Verification items for the finished model (mm, model axes). Face numbers are marked on the shaded views. A direction names the side the tool comes from. Coordinates: 2 decimals unless noted, no trailing zeros. Order: outer loops, then holes, each group sorted by start corner. A loop starts at its lowest first (then second) coordinate and runs counter-clockwise, first axis right, second up. Notation, with made-up numbers: (27, 25.5) -> (78, 25.5) arc R12 cw to (78, 32.5) -> close; hole circle Ø4 at (33, 19). An arc over 180 degrees is marked (long way). Write each question's results on one line, items separated by ' | '. Start each with the question number.
(1) Thickness scan on probe 1 along Z at (x, y) = (-0.5, -7); probe 2 along Y at (x, z) = (12.75, -7); probe 3 along Y at (x, z) = (1.25, -2). Record the ranges inside material, lowest first. Write a range as [from, to].
(2) Go/stop test with flat-tipped pins: pin 1 (1 mm diameter, centred on x = 9.5, y = -64, fed in from +Z); pin 2 (6 mm diameter, centred on x = 8.5, z = -6, fed in from +Y); pin 3 (3 mm diameter, centred on y = -14, z = 4, fed in from +X). Record where each tip stops, or that it passes through.
(3) Draft check along X on the marked faces 3, 4, 5 and 6. Enter one of: +X half, -X half, draft (parallel to the pull), parting line (faces both ways), or undercut.
(4) Set-up check for the marked faces 1 and 2: record each of +Z, -Z, +X, -X, +Y, -Y from which the full face is reachable in a straight line by a thin tool's end or side.
(5) Cross-section at A-A on y = 5.5. Enter the section's corners in (x, z), and give its area (3 significant figures).
(6) Cross-section at B-B on y = -47. Enter the section's corners in (x, z), and give its area (3 significant figures).
```python
from build123d import *

# Parameters (mm, degrees)
BOSS_EXTRUDE1_DEPTH = 12
SKETCH3_R           = 10
BOSS_EXTRUDE2_DEPTH = 75
CHAMFER1_SIZE       = 1


with BuildPart() as part:
    # Sketch1 → Boss-Extrude1 (new body)
    with BuildSketch(Plane(origin=(0, 0, 0), x_dir=(1, 0, 0), z_dir=(0, 1, 0))):
        Polygon((14, 8.082903769), (0, 16.165807537), (-14, 8.082903769), (-14, -8.082903769), (0, -16.165807537), (14, -8.082903769), align=None)
    extrude(amount=BOSS_EXTRUDE1_DEPTH)

    # Cut-Extrude1 cone 1 section (through the dimple's axis) → Cut-Extrude1 (revolve, cut)
    with BuildSketch(Plane(origin=(0, 12, 0), x_dir=(0, 0, 1), z_dir=(1, 0, 0))):
        Polygon((0, 0), (14, 0), (0, 8.082903769), align=None)
    revolve(axis=Axis((0, 12, 0), (0, -1, 0)), mode=Mode.SUBTRACT)

    # Sketch3 → Boss-Extrude2 (add)
    with BuildSketch(Plane.XZ):
        with Locations(Location((0, 0, 0), (0, 0, 270))):
            Circle(SKETCH3_R)
    extrude(amount=BOSS_EXTRUDE2_DEPTH)

    # Chamfer1
    chamfer1_edges = [part.edges().sort_by_distance(p)[0] for p in [
        (0, -75, 10),
    ]]
    chamfer(chamfer1_edges, length=CHAMFER1_SIZE)


solid = part.part
```
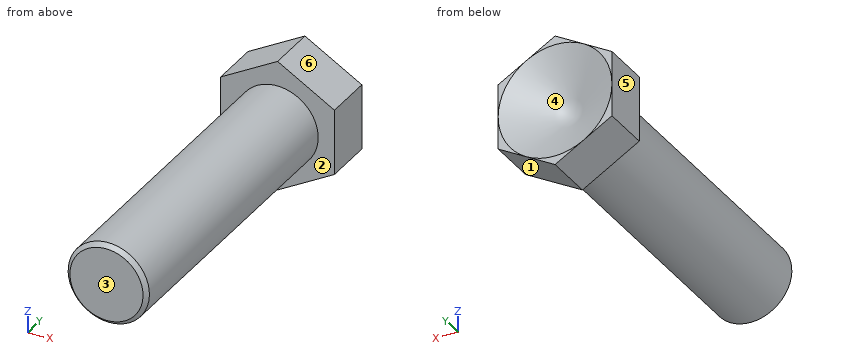
Results are:
1) probe 1: z = [-9.99, 9.99] | probe 2: y = [0, 12] | probe 3: y = [-75, 5.28]
2) pin 1: stops at z = 4.36 | pin 2: stops at y = 11.66 | pin 3: stops at x = 9.68
3) face 3: draft | face 4: undercut | face 5: -X half | face 6: +X half
4) face 1: -Z, +X, +Y, -Y | face 2: -Y
5) outline: (-14, -8.08) -> (0, -16.17) -> (14, -8.08) -> (14, 8.08) -> (0, 16.17) -> (-14, 8.08) -> close; hole circle Ø5.48 at (0, 0) | area: 655 mm2
6) outline: circle Ø20 at (0, 0) | area: 314 mm2
